```python
from build123d import *

# Parameters (mm, degrees)
F1_DEPTH = 25.4


with BuildPart() as f1:
    # F0 (on Top) → F1 (new body)
    with BuildSketch(Plane.XY):
        with BuildLine():
            ThreePointArc((-14.3874178664, 24.3026331135), (-3.6778055907, 1.497966924), (16.0707555221, 17.1422287822))
            ThreePointArc((16.0707555221, 17.1422287822), (15.6442618582, 20.8200343728), (14.3874178664, 24.3026331135))
            add(Edge.make_bspline(
                [(6.6488676301, 31.7730777763), (8.7871476467, 26.2175508691), (14.3874178664, 24.3026331135)],
                knots=[1.0830446402, 1.0830446402, 1.0830446402, 2.100651681, 2.100651681, 2.100651681], degree=2, weights=[1, 0.8733279769, 1]))
            ThreePointArc((6.6488676301, 31.7730777763), (0, 33.2129843043), (-6.6488676301, 31.7730777763))
            add(Edge.make_bspline(
                [(-14.3874178664, 24.3026331135), (-8.7871476467, 26.2175508691), (-6.6488676301, 31.7730777763)],
                knots=[1.0409409725, 1.0409409725, 1.0409409725, 2.0585480134, 2.0585480134, 2.0585480134], degree=2, weights=[1, 0.8733279769, 1]))
        make_face()
        with BuildLine():
            add(Edge.make_bspline(
                [(6.6488676301, 31.7730777763), (8.7871476467, 26.2175508691), (14.3874178664, 24.3026331135)],
                knots=[1.0830446402, 1.0830446402, 1.0830446402, 2.100651681, 2.100651681, 2.100651681], degree=2, weights=[1, 0.8733279769, 1]))
            ThreePointArc((14.3874178664, 24.3026331135), (11.1616850313, 28.7044937122), (6.6488676301, 31.7730777763))
        make_face()
        with BuildLine():
            ThreePointArc((6.6488676301, 31.7730777763), (11.1616850313, 28.7044937122), (14.3874178664, 24.3026331135))
            add(Edge.make_bspline(
                [(14.3874178664, 24.3026331135), (51.3942103362, 11.6487858527), (22.6181104936, 40.4248756132)],
                knots=[2.100651681, 2.100651681, 2.100651681, 4.7123889804, 4.7123889804, 4.7123889804], degree=2, weights=[1, 0.2618394692, 1]))
            add(Edge.make_bspline(
                [(22.6181104936, 40.4248756132), (16.5155810704, 46.5274028982), (10.0839719096, 43.0428931628), (3.6523627487, 39.5583834273), (6.6488676301, 31.7730777763)],
                knots=[4.7123889804, 4.7123889804, 4.7123889804, 6.0393094639, 6.0393094639, 7.3662299474, 7.3662299474, 7.3662299474], degree=2, weights=[1, 0.7878659738, 1, 0.7878659738, 1]))
        make_face()
        with BuildLine():
            add(Edge.make_bspline(
                [(-22.6181104936, 40.4248756132), (-51.3942103362, 11.6487858527), (-14.3874178664, 24.3026331135)],
                knots=[4.7123889804, 4.7123889804, 4.7123889804, 7.3241262797, 7.3241262797, 7.3241262797], degree=2, weights=[1, 0.2618394692, 1]))
            ThreePointArc((-14.3874178664, 24.3026331135), (-11.1616850313, 28.7044937122), (-6.6488676301, 31.7730777763))
            add(Edge.make_bspline(
                [(-6.6488676301, 31.7730777763), (-3.6523627487, 39.5583834273), (-10.0839719096, 43.0428931628), (-16.5155810704, 46.5274028982), (-22.6181104936, 40.4248756132)],
                knots=[2.0585480134, 2.0585480134, 2.0585480134, 3.3854684969, 3.3854684969, 4.7123889804, 4.7123889804, 4.7123889804], degree=2, weights=[1, 0.7878659738, 1, 0.7878659738, 1]))
        make_face()
        with BuildLine():
            ThreePointArc((-6.6488676301, 31.7730777763), (-11.1616850313, 28.7044937122), (-14.3874178664, 24.3026331135))
            add(Edge.make_bspline(
                [(-14.3874178664, 24.3026331135), (-8.7871476467, 26.2175508691), (-6.6488676301, 31.7730777763)],
                knots=[1.0409409725, 1.0409409725, 1.0409409725, 2.0585480134, 2.0585480134, 2.0585480134], degree=2, weights=[1, 0.8733279769, 1]))
        make_face()
    extrude(amount=F1_DEPTH)


solid = f1.part
```
Geometry check sheet. Reference: the model listing, model coordinates, mm. Coordinates: 2 decimals unless noted, no trailing zeros. Order: outer loops, then holes, each group sorted by start corner. A loop starts at its lowest first (then second) coordinate and runs counter-clockwise, first axis right, second up. Notation, with made-up numbers: M -8.75,79.5 L 20.25,79.5 A20 cw 20.25,85.5 Z; hole C 5.25,-33 d1. An arc over 180 degrees is marked long. One line per question, with ' | ' between items. Start each with the question number.
Item 1: Material ranges on L1, parallel to X at y = 37.5, z = 1.5; L2, parallel to X at y = 42, z = 23.5; L3, parallel to Y at x = 0.5, z = 16, recorded low to high. Write a range as [from, to].
Item 2: Cross-section at B-B on y = 8. Enter the section's corners in (x, z), then the cut area to 3 significant figures.
Item 3: Cross-section at A-A on x = 0. Enter the section's corners in (y, z).
Item 4: Gauge pin test, flat ends, axial feed: pin 1 (12 mm diameter, centred on y = 21, z = 12.5, fed in from +X); pin 2 (1.5 mm diameter, centred on x = 2, z = 11.5, fed in from -Y); pin 3 (4 mm diameter, centred on x = 20.5, z = 22, fed in from -Y). Record the tip position at first contact, or that the pin passes through.
Findings:
1) L1: x = [-24.82, -6.08], [6.08, 24.82] | L2: x = [-20.71, -8.6], [8.6, 20.71] | L3: y = [1.08, 33.21]
2) outline: M -13.22,0 L 13.22,0 L 13.22,25.4 L -13.22,25.4 Z | area: 671 mm²
3) outline: M 1.07,0 L 33.21,0 L 33.21,25.4 L 1.07,25.4 Z
4) pin 1: stops at x = 24.67 | pin 2: stops at y = 1.12 | pin 3: stops at y = 23.73
